For this review, take the finished solid that the model builds, in its own axes (mm). Coordinates: 2 decimals unless noted, no trailing zeros. Write each loop counter-clockwise with the first axis right and the second up, starting at its lowest first coordinate (ties: lowest second). Pieces come first, ordered by that corner, then holes. Notation, with made-up numbers: (-20, 52) -> (27, 52) arc R15 cw to (27, 60) -> close; hole circle Ø10 at (-12, 64). An arc over 180 degrees is marked (long way). Put each result on its own line as item: value. Start each with the question number.
Item 1: Consider section A-A on z = 279. Give the boundary of the cut face in (x, y).
Item 2: Insertion check: P1, Ø5.5, axis at y = 0, z = 405, coming from the +X side; P2, Ø8, axis at x = 3.5, y = 2, coming from the +Z side. Each pin has a flat end and moves straight along its axis. Give the tip position at first contact, or say it passes through.
Item 3: To check wall thickness, follow L1, parallel to Z at x = -9.3, y = 0; L2, parallel to Z at x = 0.25, y = 8.5; L3, parallel to X at y = 5.25, z = 354. State the ranges of each line that lie inside material, in increasing order.
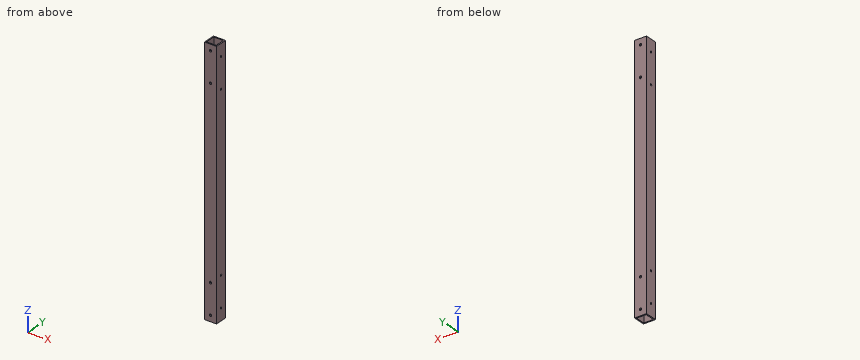
Autodesk Inventor part; units mm, degrees
ref_plane "YZ Plane" through (0, 0, 0) normal (1, 0, 0) x (0, 1, 0)
ref_plane "XZ Plane" through (0, 0, 0) normal (0, 1, 0) x (-1, 0, 0)
ref_plane "XY Plane" through (0, 0, 0) normal (0, 0, 1) x (1, 0, 0)
sketch "スケッチ1" plane through (0, 0, 0) normal (0, 0, 1) x (1, 0, 0)
  line L0 (10, -10) -> (-10, -10)
  line L1 (-10, -10) -> (-10, 10)
  line L2 (-10, 10) -> (10, 10)
  line L3 (10, 10) -> (10, -10)
  line L4 (10, -10) -> (-10, 10) construction
  line L5 (-10, -10) -> (10, 10) construction
  line L6 (8, 8) -> (-8, 8)
  line L7 (-8, 8) -> (-8, -8)
  line L8 (-8, -8) -> (8, -8)
  line L9 (8, -8) -> (8, 8)
  point P0 (0, 0)
  dimension "d0" = 20
  dimension "d1" = 20
  dimension "d2" = 2
extrude "押し出し1" add sketch "スケッチ1" along normal blind 425
sketch "スケッチ2" plane through (-10, 10, 0) normal (0, 1, 0) x (1, 0, 0)
  line L0 (10, 0) -> (10, -425)
  line L1 (2, -425) -> (18, -425)
  line L2 (20, 0) -> (0, 0)
  point P0 (10, -415)
  point P1 (10, -365)
  point P2 (10, -60)
  point P3 (10, -10)
  dimension "d5" = 10
  dimension "d6" = 50
  dimension "d7" = 50
  dimension "d9" = 10
hole "穴1" at (0, 10, 415) at (0, 10, 365) at (0, 10, 60) at (0, 10, 10) direction (0, -1, 0) diameter 4 end through all
sketch "スケッチ3" plane through (10, -10, 0) normal (1, 0, 0) x (0, 0, -1)
  line L0 (0, 10) -> (-425, 10)
  line L1 (-425, 20) -> (-425, 0)
  line L2 (0, 0) -> (0, 20)
  point P0 (-405, 10)
  point P1 (-355, 10)
  point P2 (-20, 10)
  point P3 (-70, 10)
  dimension "d17" = 20
  dimension "d18" = 50
  dimension "d19" = 20
  dimension "d20" = 50
hole "穴2" at (10, 0, 405) at (10, 0, 355) at (10, 0, 20) at (10, 0, 70) direction (-1, 0, 0) diameter 3.3 end through all
properties part number "aaa_small_kaku_2020_tka"
Return value:
1. outline: (-10, -10) -> (10, -10) -> (10, 10) -> (-10, 10) -> close; hole (-8, -8) -> (8, -8) -> (8, 8) -> (-8, 8) -> close
2. P1: x = 10
2. P2: through
3. L1: 0 to 18.35, 21.65 to 68.35, 71.65 to 353.35, 356.65 to 403.35, 406.65 to 425
3. L2: 0 to 8.02, 11.98 to 58.02, 61.98 to 363.02, 366.98 to 413.02, 416.98 to 425
3. L3: -10 to -8, 8 to 10
